from build123d import *

# Parameters (mm, degrees)
SKETCH1_W                = 20
SKETCH1_H                = 11
BOSS_EXTRUDE1_DEPTH      = 4
SKETCH2_W                = 30.8
SKETCH2_H                = 12.5
BOSS_EXTRUDE2_DEPTH      = 1
F_3_0_3_DIAMETER_HOLE1_D = 3


with BuildPart() as part:
    # Sketch1 → Boss-Extrude1 (new body)
    with BuildSketch(Plane.XY):
        Rectangle(SKETCH1_W, SKETCH1_H)
    extrude(amount=BOSS_EXTRUDE1_DEPTH)

    # Sketch2 → Boss-Extrude2 (add)
    with BuildSketch(Plane.XY.offset(4)):
        Rectangle(SKETCH2_W, SKETCH2_H)
    extrude(amount=BOSS_EXTRUDE2_DEPTH)

    # Ø3.0 (3) Diameter Hole1 (through all)
    with Locations(Plane.XY.offset(5)):
        with Locations((-12.65, 0), (12.65, 0)):
            Hole(F_3_0_3_DIAMETER_HOLE1_D / 2)


solid = part.part
Check sheet for the modelled part. Datum: model origin and axes. Units: mm. A direction names the side the tool comes from. Give positions to 0.01 mm unless a question says otherwise; leave off trailing zeros. Order: outer loops, then holes, each group sorted by start corner. A loop starts at its lowest first (then second) coordinate and runs counter-clockwise, first axis right, second up. Notation, with made-up numbers: M 31.5,-14 L 50.5,-14 A22 cw 50.5,4 Z; hole C 81,-28.75 d2. An arc over 180 degrees is marked long. Answer as CSV lines item,"result". Start each with the question number.
Item 1: Gauge pin test, flat ends, axial feed: P1, Ø5, axis at x = 12.65, y = 0, coming from the -Z side; P2, Ø3, axis at x = -1, z = 1.5, coming from the -Y side; P3, Ø2, axis at y = -1, z = 1, coming from the -X side. Record the tip position at first contact, or that the pin passes through.
Item 2: Tool access check on faces 1 (the face through (0, -5.5, 2)), 2 (the face through (-10, 0, 2)), 3 (the face through (0, 5.5, 2)). Record the directions out of +Z, -Z, +X, -X, +Y, -Y that give a thin tool (end or side, any length) a straight path to the whole face; none if there is none.
Item 3: Cross-section at A-A on x = 12.65. Enter the section's corners in (y, z).
Item 4: Cross-section at C-C on y = 3. Enter the section's corners in (x, z).
Item 5: Cross-section at D-D on x = 0. Enter the section's corners in (y, z), plus the area to 3 significant figures.
Item 6: Mould release check, pull along Y, two halves, no side actions. Record for faces 4 (the face through (-11.15, 0.07, 4.49)), 5 (the face through (-0.2, -6.25, 4.5)), 6 (the face through (10, 0, 2)): +Y half, -Y half, draft (parallel to the pull), parting line (faces both ways), or undercut.
Item 7: Cross-section at B-B on y = 0. Enter the section's corners in (x, z).
Item 8: Thickness scan on line 1 (Y direction, x = 12.65, z = 4.45); line 2 (Z direction, x = -13.5, y = -4.75); line 3 (X direction, y = -4.25, z = 0.75). Record the ranges inside material, lowest first. Write a range as [from, to].
Established:
1,P1,"stops at z = 4"
1,P2,"stops at y = -5.5"
1,P3,"stops at x = -10"
2,face 1,"-Z, +X, -X, -Y"
2,face 2,"-Z, -X, +Y, -Y"
2,face 3,"-Z, +X, -X, +Y"
3,outline,"M -6.25,4 L -1.5,4 L -1.5,5 L -6.25,5 Z; M 1.5,4 L 6.25,4 L 6.25,5 L 1.5,5 Z"
4,outline,"M -15.4,4 L -10,4 L -10,0 L 10,0 L 10,4 L 15.4,4 L 15.4,5 L -15.4,5 Z"
5,outline,"M -6.25,4 L -5.5,4 L -5.5,0 L 5.5,0 L 5.5,4 L 6.25,4 L 6.25,5 L -6.25,5 Z"
5,area,"56.5 mm^2"
6,face 4,"undercut"
6,face 5,"-Y half"
6,face 6,"draft"
7,outline,"M -15.4,4 L -14.15,4 L -14.15,5 L -15.4,5 Z; M -11.15,4 L -10,4 L -10,0 L 10,0 L 10,4 L 11.15,4 L 11.15,5 L -11.15,5 Z; M 14.15,4 L 15.4,4 L 15.4,5 L 14.15,5 Z"
8,line 1,"y = [-6.25, -1.5], [1.5, 6.25]"
8,line 2,"z = [4, 5]"
8,line 3,"x = [-10, 10]"
